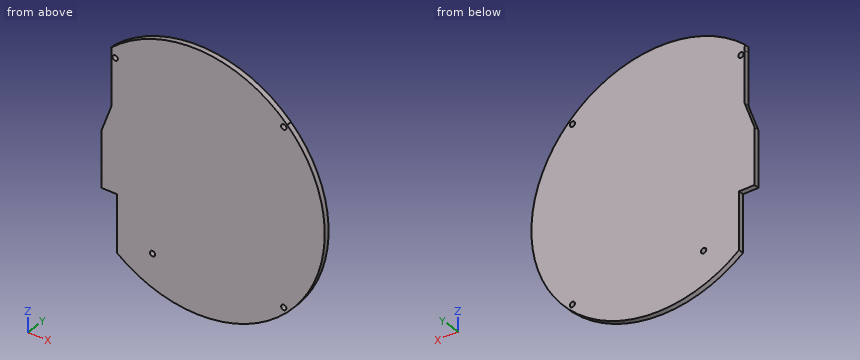
Autodesk Inventor part; units mm, degrees
ref_plane "YZ Plane" through (0, 0, 0) normal (1, 0, 0) x (0, 1, 0)
ref_plane "XZ Plane" through (0, 0, 0) normal (0, 1, 0) x (-1, 0, 0)
ref_plane "XY Plane" through (0, 0, 0) normal (0, 0, 1) x (1, 0, 0)
sketch "Sketch1" plane through (0, 0, 0) normal (0, 1, 0) x (-1, 0, 0)
  line L0 (0, 0) -> (0, -51.9)
  line L1 (0, -51.9) -> (39.53, -51.9)
  line L2 (0, 0) -> (53.1, 0)
  line L3 (0, 0) -> (50.2, 0)
  line L4 (50.2, 0) -> (50.2, -14.6)
  line L5 (50.2, 0) -> (64.8, 0) construction
  line L6 (50.2, -14.6) -> (53.1008, -22.6003)
  line L7 (50.2, -14.6) -> (58.71, -14.6) construction
  line L8 (53.1008, -22.6003) -> (53.1008, -38.4903)
  line L9 (53.1008, -38.4903) -> (48.6508, -38.4903)
  line L10 (48.6508, -38.4903) -> (39.53, -51.9)
  dimension "d0" = 51.9
  dimension "d1" = 39.53
  dimension "d9" = 50.2
  dimension "d10" = 14.6
  dimension "d11" = 90
  dimension "d12" = 8.51
  dimension "d13" = 70.07
  dimension "d14" = 15.89
  dimension "d17" = 4.45
extrude "Extrusion1" add sketch "Sketch1" along normal blind 1.5
sketch "Sketch2" plane through (0, 1.5, 0) normal (0, 1, 0) x (1, 0, 0)
  circle A0 centre (-1, 1) radius 0.75
  point P0 (0, 0)
  dimension "d22" = 1.5
extrude "Extrusion2" cut sketch "Sketch2" against normal blind 10
sketch "Sketch3" plane through (0, 1.5, 0) normal (0, 1, 0) x (1, 0, 0)
  line L0 (0, 0) -> (0, 51.9)
  line L1 (0, 51.9) -> (-39.53, 51.9)
  circle A0 centre (-1, 50.9) radius 0.75
  dimension "d27" = 1.5
extrude "Extrusion3" cut sketch "Sketch3" against normal blind 10
sketch "Sketch4" plane through (0, 1.5, 0) normal (0, 1, 0) x (1, 0, 0)
  circle A0 centre (-49.2, 1) radius 0.75
  line L0 (-39.53, 51.9) -> (-48.6508, 38.4903)
  circle A1 centre (-38.53, 50.9) radius 0.75
  point P0 (0, 0)
  point P1 (-50.2, 0)
  dimension "d32" = 1.5
  dimension "d35" = 1.5
extrude "Extrusion4" cut sketch "Sketch4" against normal blind 10
sketch "Sketch5" plane through (0, 1.5, 0) normal (0, 1, 0) x (1, 0, 0)
  line L0 (0, 0) -> (0, 51.9)
  line L1 (0, 25.95) -> (-25.95, 25.95)
  arc A0 (-50.3282, -1.4419) -> (-48.6508, 54.7474) centre (-25.95, 25.95) ccw
  line L2 (-39.53, 51.9) -> (-48.6508, 38.4903)
  line L3 (-48.6508, 38.4903) -> (-48.6508, 54.7474)
  line L4 (-39.53, 51.9) -> (0, 51.9)
  line L5 (0, 0) -> (0, 51.9)
  line L6 (-50.2, 0) -> (0, 0)
  line L7 (0, 0) -> (-50.2, 0)
  line L8 (-50.2, 0) -> (-50.3282, -1.4419)
  point P0 (-0.0422, 51.9)
  point P1 (0, 0.0422)
  point P2 (0, 51.8578)
  point P3 (-0.0422, 0)
  dimension "d38" = 25.95
  dimension "d39" = 36.669
extrude "Extrusion5" add sketch "Sketch5" against normal blind 1.5 contours A0 L8 L6 | L4 L2 L3 A0 | L0 A0
properties part number "CaseCover"
Work out the finished part from the listing and answer in its coordinate system (mm). Give positions to 0.01 mm unless a question says otherwise; leave off trailing zeros. Write each loop counter-clockwise with the first axis right and the second up, starting at its lowest first coordinate (ties: lowest second). Pieces come first, ordered by that corner, then holes. Notation, with made-up numbers: (-36.5, 73.25) - (-32.5, 73.25) arc R14 cw to (-32.5, 84.25) - close; hole circle Ø4 at (15.5, 0.5). An arc over 180 degrees is marked (long way). Use one line per item in the form item = value.
1. A cutting plane is placed at B-B (z = -5). Write down the section's boundary in (x, y) (3 decimals), and give its area (3 significant figures).
Filled in:
outline = (-50.2, 0) - (4.145, 0) - (4.145, 1.5) - (-50.2, 1.5) - close
area = 81.5 mm^2
2. Consider L1, parallel to X at y = 0.4, z = -50.9; L2, parallel to X at y = 0.55, z = -1; L3, parallel to Z at x = -1, y = 1. Determine where each line is inside the solid, lowest interval first.
Filled in:
L1 = -48.65 to -39.28, -37.78 to -1.75, -0.25 to 0.92
L2 = -50.2 to -49.95, -48.45 to -1.75, -0.25 to 0.92
L3 = -52.82 to -51.65, -50.15 to -1.75, -0.25 to 0.92
3. A cutting plane is placed at C-C (x = -42). Write down the section's boundary in (y, z).
Filled in:
outline = (0, -58.92) - (1.5, -58.92) - (1.5, 7.02) - (0, 7.02) - close
4. A cutting plane is placed at A-A (y = 0.6). Write down the section's boundary in (x, z).
Filled in:
outline = (-53.1, -38.49) - (-48.65, -38.49) - (-48.65, -54.75) arc R36.67 ccw to (-0.04, -51.9) - (0, -51.9) - (0, -51.86) arc R36.67 ccw to (0, -0.04) - (0, 0) - (-0.04, 0) arc R36.67 ccw to (-50.33, 1.44) - (-50.2, 0) - (-50.2, -14.6) - (-53.1, -22.6) - close; hole circle Ø1.5 at (-49.2, -1); hole circle Ø1.5 at (-38.53, -50.9); hole circle Ø1.5 at (-1, -50.9); hole circle Ø1.5 at (-1, -1)
